```python
from build123d import *

# Parameters (mm, degrees)
SKETCH2_W           = 10
SKETCH2_H           = 13
SKETCH2_R           = 1.25
BOSS_EXTRUDE1_DEPTH = 5
FILLET1_R           = 1
SKETCH3_R           = 0.7
CUT_EXTRUDE1_DEPTH  = 3


with BuildPart() as part:
    # Sketch2 → Boss-Extrude1 (new body)
    with BuildSketch(Plane.XY):
        Rectangle(SKETCH2_W, SKETCH2_H)
        with Locations((-2.5, 4.5)):
            Circle(SKETCH2_R, mode=Mode.SUBTRACT)
        with Locations((2.5, 4.5)):
            Circle(SKETCH2_R, mode=Mode.SUBTRACT)
        with Locations((2.5, 1.5)):
            Circle(SKETCH2_R, mode=Mode.SUBTRACT)
        with Locations((2.5, -1.5)):
            Circle(SKETCH2_R, mode=Mode.SUBTRACT)
        with Locations((2.5, -4.5)):
            Circle(SKETCH2_R, mode=Mode.SUBTRACT)
        with Locations((-2.5, 1.5)):
            Circle(SKETCH2_R, mode=Mode.SUBTRACT)
        with Locations((-2.5, -1.5)):
            Circle(SKETCH2_R, mode=Mode.SUBTRACT)
        with Locations((-2.5, -4.5)):
            Circle(SKETCH2_R, mode=Mode.SUBTRACT)
        Circle(SKETCH2_R, mode=Mode.SUBTRACT)
    extrude(amount=BOSS_EXTRUDE1_DEPTH)

    # Fillet1
    fillet1_edges = [part.edges().sort_by_distance(p)[0] for p in [
        (-5, 0, 0),
        (5, 0, 0),
        (5, 0, 5),
        (-5, 0, 5),
    ]]
    fillet(fillet1_edges, radius=FILLET1_R)

    # Sketch3 → Cut-Extrude1 (cut)
    with BuildSketch(Plane(origin=(0, 6.5, 0), x_dir=(1, 0, 0), z_dir=(0, 1, 0))):
        with Locations((0, -2.5)):
            Circle(SKETCH3_R)
    cut_extrude1 = extrude(amount=-CUT_EXTRUDE1_DEPTH, mode=Mode.SUBTRACT)

    # Mirror1: Cut-Extrude1 across plane
    add(cut_extrude1.mirror(Plane.ZX), mode=Mode.SUBTRACT)


solid = part.part
```
Model file for the job. Use its own axes, mm. A direction names the side the tool comes from. Coordinates: 2 decimals unless noted, no trailing zeros. Order: outer loops, then holes, each group sorted by start corner. A loop starts at its lowest first (then second) coordinate and runs counter-clockwise, first axis right, second up. Notation, with made-up numbers: (49, 70) -> (89, 70) arc R19 ccw to (89, 81) -> close; hole circle Ø9 at (4.25, -5.5). An arc over 180 degrees is marked (long way). Answer as a JSON object with one key per item and string values. Group by question number.
1) Cut at C-C, the plane y = 0. Write the cut outline in (x, z).
2) Pull direction X, two halves, no side cores. Call faces 1 (the face through (4.715, 0.091, 0.301)), 2 (the face through (-1.923, 3.391, 2.465)), 3 (the face through (0, 6.5, 1)): +X half, -X half, draft (parallel to the pull), parting line (faces both ways), or undercut.
3) Flat gauge pins, fed straight in: pin 1 (1.5 mm diameter, centred on x = 0, y = 0, fed in from -Z); pin 2 (1.1 mm diameter, centred on x = 0, z = 2.5, fed in from -Y). Where does each tip first touch, or does it go through?
4) Cut at D-D, the plane x = 2.5. Write the cut outline in (y, z), then the cut area to 3 significant figures.
5) Drill centre lines: L1, parallel to Y at x = 2.5, z = 3.6; L2, parallel to X at y = 2.5, z = 0.65; L3, parallel to X at y = -5.4, z = 2.5. Where is each one in solid material? Low to high.
6) Cut at B-B, the plane x = 0. Write the cut outline in (y, z), then the cut area to 3 significant figures.
7) Cut at A-A, the plane y = -5.5. Write the cut outline in (x, z).
8) Which spindle directions (+Z, -Z, +X, -X, +Y, -Y) get a long thin tool onto all of the face, cutting with end or side? Do faces 4 (the face through (0, -3.5, 2)), 5 (the face through (0, 3.5, 2)), 6 (the face through (3.69, -1.12, 2.46)). Say none if no direction does.
Check values:
{
 "1": {"outline": "(-5, 1) arc R1 ccw to (-4, 0) -> (-1.25, 0) -> (-1.25, 5) -> (-4, 5) arc R1 ccw to (-5, 4) -> close; (1.25, 0) -> (4, 0) arc R1 ccw to (5, 1) -> (5, 4) arc R1 ccw to (4, 5) -> (1.25, 5) -> close"},
 "2": {"face 1": "+X half", "face 2": "undercut", "face 3": "draft"},
 "3": {"pin 1": "passes through", "pin 2": "stops at y = -3.5"},
 "4": {"outline": "(-6.5, 0) -> (-5.75, 0) -> (-5.75, 5) -> (-6.5, 5) -> close; (-3.25, 0) -> (-2.75, 0) -> (-2.75, 5) -> (-3.25, 5) -> close; (-0.25, 0) -> (0.25, 0) -> (0.25, 5) -> (-0.25, 5) -> close; (2.75, 0) -> (3.25, 0) -> (3.25, 5) -> (2.75, 5) -> close; (5.75, 0) -> (6.5, 0) -> (6.5, 5) -> (5.75, 5) -> close", "area": "15.0 mm²"},
 "5": {"L1": "y = -6.5 to -5.75, -3.25 to -2.75, -0.25 to 0.25, 2.75 to 3.25, 5.75 to 6.5", "L2": "x = -4.94 to -3.25, -1.75 to 1.75, 3.25 to 4.94", "L3": "x = -5 to -3.37, -1.63 to -0.7, 0.7 to 1.63, 3.37 to 5"},
 "6": {"outline": "(-6.5, 0) -> (-1.25, 0) -> (-1.25, 5) -> (-6.5, 5) -> (-6.5, 3.2) -> (-3.5, 3.2) -> (-3.5, 1.8) -> (-6.5, 1.8) -> close; (1.25, 0) -> (6.5, 0) -> (6.5, 1.8) -> (3.5, 1.8) -> (3.5, 3.2) -> (6.5, 3.2) -> (6.5, 5) -> (1.25, 5) -> close", "area": "44.1 mm²"},
 "7": {"outline": "(-5, 1) arc R1 ccw to (-4, 0) -> (-3.25, 0) -> (-3.25, 5) -> (-4, 5) arc R1 ccw to (-5, 4) -> close; (-1.75, 0) -> (1.75, 0) -> (1.75, 5) -> (-1.75, 5) -> close; (3.25, 0) -> (4, 0) arc R1 ccw to (5, 1) -> (5, 4) arc R1 ccw to (4, 5) -> (3.25, 5) -> close; hole circle Ø1.4 at (0, 2.5)"},
 "8": {"face 4": "-Y", "face 5": "+Y", "face 6": "+Z, -Z"}
}
